```python
from build123d import *

# Parameters (mm, degrees)
SKETCH1_W           = 45
SKETCH1_H           = 70
BOSS_EXTRUDE1_DEPTH = 3
SKETCH2_R           = 10.95
SKETCH2_W           = 24
SKETCH2_H           = 35
CUT_EXTRUDE1_DEPTH  = 4
FILLET1_R           = 4
SKETCH4_W           = 10
SKETCH4_H           = 3
BOSS_EXTRUDE3_DEPTH = 3
SKETCH3_W           = 3
SKETCH3_H           = 14
BOSS_EXTRUDE2_DEPTH = 3


with BuildPart() as part:
    # Sketch1 → Boss-Extrude1 (new body)
    with BuildSketch(Plane.XY):
        Rectangle(SKETCH1_W, SKETCH1_H)
    extrude(amount=BOSS_EXTRUDE1_DEPTH)

    # Sketch2 → Cut-Extrude1 (cut, through all)
    with BuildSketch(Plane.XY.offset(3)):
        with Locations((0, 16)):
            Circle(SKETCH2_R)
        with Locations((0, -17.5)):
            Rectangle(SKETCH2_W, SKETCH2_H)
    extrude(amount=-CUT_EXTRUDE1_DEPTH, mode=Mode.SUBTRACT)

    # Fillet1
    fillet1_edges = [part.edges().sort_by_distance(p)[0] for p in [
        (12, 0, 1.5),
        (-12, 0, 1.5),
    ]]
    fillet(fillet1_edges, radius=FILLET1_R)

    # Sketch4 → Boss-Extrude3 (add)
    with BuildSketch(Plane.XY.offset(3)):
        with Locations((-10, 36.5)):
            Rectangle(SKETCH4_W, SKETCH4_H)
        with Locations((10, 36.5)):
            Rectangle(SKETCH4_W, SKETCH4_H)
    extrude(amount=-BOSS_EXTRUDE3_DEPTH)

    # Sketch3 → Boss-Extrude2 (add)
    with BuildSketch(Plane(origin=(0, 0, 0), x_dir=(-1, 0, 0), z_dir=(0, 0, -1))):
        with Locations((24, 0)):
            Rectangle(SKETCH3_W, SKETCH3_H)
        with Locations((24, 28)):
            Rectangle(SKETCH3_W, SKETCH3_H)
        with Locations((24, -28)):
            Rectangle(SKETCH3_W, SKETCH3_H)
        with Locations((-24, 14)):
            Rectangle(SKETCH3_W, SKETCH3_H)
        with Locations((-24, -14)):
            Rectangle(SKETCH3_W, SKETCH3_H)
    extrude(amount=-BOSS_EXTRUDE2_DEPTH)


solid = part.part
```
Could you check a few things on this model? Use its own coordinates, in mm. A direction names the side the tool comes from. Round coordinates to 2 decimals unless told otherwise and drop trailing zeros. Write each loop counter-clockwise with the first axis right and the second up, starting at its lowest first coordinate (ties: lowest second). Pieces come first, ordered by that corner, then holes. Notation, with made-up numbers: M 76.25,12 L 105.25,12 A22 ccw 105.25,37 Z; hole C 64,13 d2. An arc over 180 degrees is marked long. Answer in a Markdown table with one row per item. Add a question column.
Q1. If I drill on line 1 (X direction, y = -10, z = 1.65); line 2 (Y direction, x = 0, z = 2.05); line 3 (Y direction, x = -4, z = 0.45), over which ranges is the centre line in solid material (lowest first)? Write a range as from..to.
Q2. If we mould it in two halves opening along Y, with no side actions, what happens to faces 1 (the flat face through (-22.5, -14, 1)), 2 (the flat face through (-22.5, 14, 1)), 3 (the flat face through (24, 21, 1)), 4 (the flat face through (24, -21, 1))? For each: +Y half, -Y half, draft (parallel to the pull), parting line (faces both ways), or undercut.
Q3. On a 3-axis mill with a long thin cutter (end or side, diameter ignored), from which of +Z, -Z, +X, -X, +Y, -Y can I reach the whole of each face in a straight line? I mean faces 5 (the flat face through (-20, 35, 1)), 6 (the flat face through (-24, 7, 1)), 7 (the flat face through (-5, 36, 2)), 8 (the flat face through (24, 7, 1)). Say none if no direction works.
Q4. Will these pins go through, and if not, where does the flat tip stop? pin 1 Ø1.5 at (y, z) = (36.5, 1.5) entering from +X; pin 2 Ø1.5 at (y, z) = (36.5, 2) entering from -X; pin 3 Ø1 at (x, z) = (4, 2) entering from +Y.
Q5. Imagine slicing it at C-C (x = 21). Please give me the cut outline in (y, z).
Q6. Imagine slicing it at B-B (y = 16). Please give me the cut outline in (x, z).
Q7. Imagine slicing it at A-A (x = 0). Please give me the cut outline in (y, z), then the cut area to 3 significant figures.
Values:
| question | item | result |
|---|---|---|
| 1 | line 1 | -22.5..-12, 12..25.5 |
| 1 | line 2 | 0..5.05, 26.95..35 |
| 1 | line 3 | 0..5.81, 26.19..35 |
| 2 | face 1 | undercut |
| 2 | face 2 | undercut |
| 2 | face 3 | +Y half |
| 2 | face 4 | -Y half |
| 3 | face 5 | +Z, -Z, -X, +Y |
| 3 | face 6 | +Z, -Z, -X |
| 3 | face 7 | +Z, -Z, +Y |
| 3 | face 8 | +Z, -Z, +X |
| 4 | pin 1 | x = 15 |
| 4 | pin 2 | x = -15 |
| 4 | pin 3 | y = 35 |
| 5 | outline | M -35,0 L 35,0 L 35,3 L -35,3 Z |
| 6 | outline | M -22.5,0 L -10.95,0 L -10.95,3 L -22.5,3 Z; M 10.95,0 L 25.5,0 L 25.5,3 L 10.95,3 Z |
| 7 | outline | M 0,0 L 5.05,0 L 5.05,3 L 0,3 Z; M 26.95,0 L 35,0 L 35,3 L 26.95,3 Z |
| 7 | area | 39.3 mm^2 |
